```python
from build123d import *

# Parameters (mm, degrees)
SKETCH1_W           = 4.2
SKETCH1_H           = 10.1
SKETCH1_W_2         = 20.4
SKETCH1_H_2         = 14.2
BOSS_EXTRUDE1_DEPTH = 5.95
SKETCH2_R           = 5.1
BOSS_EXTRUDE2_DEPTH = 8.7


with BuildPart() as part:
    # Sketch1 → Boss-Extrude1 (new, symmetric)
    with BuildSketch(Plane(origin=(0, 0, 0), x_dir=(1, 0, 0), z_dir=(0, 1, 0))):
        with Locations((-12.3, 0)):
            Rectangle(SKETCH1_W, SKETCH1_H)
        Rectangle(SKETCH1_W_2, SKETCH1_H_2)
    extrude(amount=BOSS_EXTRUDE1_DEPTH, both=True)

    # Sketch2 → Boss-Extrude2 (add)
    with BuildSketch(Plane(origin=(10.2, 0, 0), x_dir=(0, 0, -1), z_dir=(1, 0, 0))):
        Circle(SKETCH2_R)
    extrude(amount=BOSS_EXTRUDE2_DEPTH)


solid = part.part
```
Geometry check sheet. Reference: the model listing, model coordinates, mm. A direction names the side the tool comes from. Round coordinates to 2 decimals unless told otherwise and drop trailing zeros. Loops run counter-clockwise (first coordinate to the right, second up) from the corner with the lowest first, then second, coordinate; pieces in that order, holes last. Notation, with made-up numbers: (-39.5, 14.25) -> (18.5, 14.25) arc R22 ccw to (18.5, 43.25) -> close; hole circle Ø8 at (-3.5, -18.75). An arc over 180 degrees is marked (long way). Use a Markdown table: item, result.
(1) Sectioned sample at A-A (y = 0). Enter the section's corners in (x, z), then the cut area to 3 significant figures.
Calculated:
| item | result |
|---|---|
| outline | (-14.4, -5.05) -> (-10.2, -5.05) -> (-10.2, -7.1) -> (10.2, -7.1) -> (10.2, -5.1) -> (18.9, -5.1) -> (18.9, 5.1) -> (10.2, 5.1) -> (10.2, 7.1) -> (-10.2, 7.1) -> (-10.2, 5.05) -> (-14.4, 5.05) -> close |
| area | 421 mm² |
(2) Sectioned sample at D-D (z = 0). Enter the section's corners in (x, y).
Calculated:
| item | result |
|---|---|
| outline | (-14.4, -5.95) -> (10.2, -5.95) -> (10.2, -5.1) -> (18.9, -5.1) -> (18.9, 5.1) -> (10.2, 5.1) -> (10.2, 5.95) -> (-14.4, 5.95) -> close |
(3) Scan lines: probe 1 along X at (y, z) = (-5.25, 5.25); probe 2 along Z at (x, y) = (12.5, 0.75); probe 3 along X at (y, z) = (-3, 4.25). Record each from-to range of solid material in increasing order.
Calculated:
| item | result |
|---|---|
| probe 1 | -10.2 to 10.2 |
| probe 2 | -5.04 to 5.04 |
| probe 3 | -14.4 to 10.2 |
(4) Go/stop test with flat-tipped pins: P1, Ø1.6, axis at y = -2.5, z = -6, coming from the -X side; P2, Ø2, axis at x = -11.5, y = -1, coming from the -Z side; P3, Ø2, axis at x = -12.5, y = -2, coming from the +Z side. Record where each tip stops, or that it passes through.
Calculated:
| item | result |
|---|---|
| P1 | x = -10.2 |
| P2 | z = -5.05 |
| P3 | z = 5.05 |
(5) Sectioned sample at C-C (x = -11). Enter the section's corners in (y, z).
Calculated:
| item | result |
|---|---|
| outline | (-5.95, -5.05) -> (5.95, -5.05) -> (5.95, 5.05) -> (-5.95, 5.05) -> close |
(6) Set-up check for faces 1 (the flat face through (10.2, 5.4, 0.1)), 2 (the flat face through (-10.2, 0, 6)), 3 (the flat face through (-10.2, 0, -6)): record each of +Z, -Z, +X, -X, +Y, -Y from which the full face is reachable in a straight line by a thin tool's end or side.
Calculated:
| item | result |
|---|---|
| face 1 | +X |
| face 2 | +Z, -X, +Y, -Y |
| face 3 | -Z, -X, +Y, -Y |
(7) Sectioned sample at B-B (z = -4.5). Enter the section's corners in (x, y).
Calculated:
| item | result |
|---|---|
| outline | (-14.4, -5.95) -> (10.2, -5.95) -> (10.2, -2.4) -> (18.9, -2.4) -> (18.9, 2.4) -> (10.2, 2.4) -> (10.2, 5.95) -> (-14.4, 5.95) -> close |
